Geometry check sheet. Reference: drawing and pictorial views, mm from the part's lowest x, y, z. Give positions to 0.01 mm unless a question says otherwise; leave off trailing zeros. Order: outer loops, then holes, each group sorted by start corner. A loop starts at its lowest first (then second) coordinate and runs counter-clockwise, first axis right, second up. Notation, with made-up numbers: M 89,43 L 146,43 A26 ccw 146,68 Z; hole C 80,40 d7. An arc over 180 degrees is marked long. Answer as a JSON object with one key per item and string values. Group by question number.
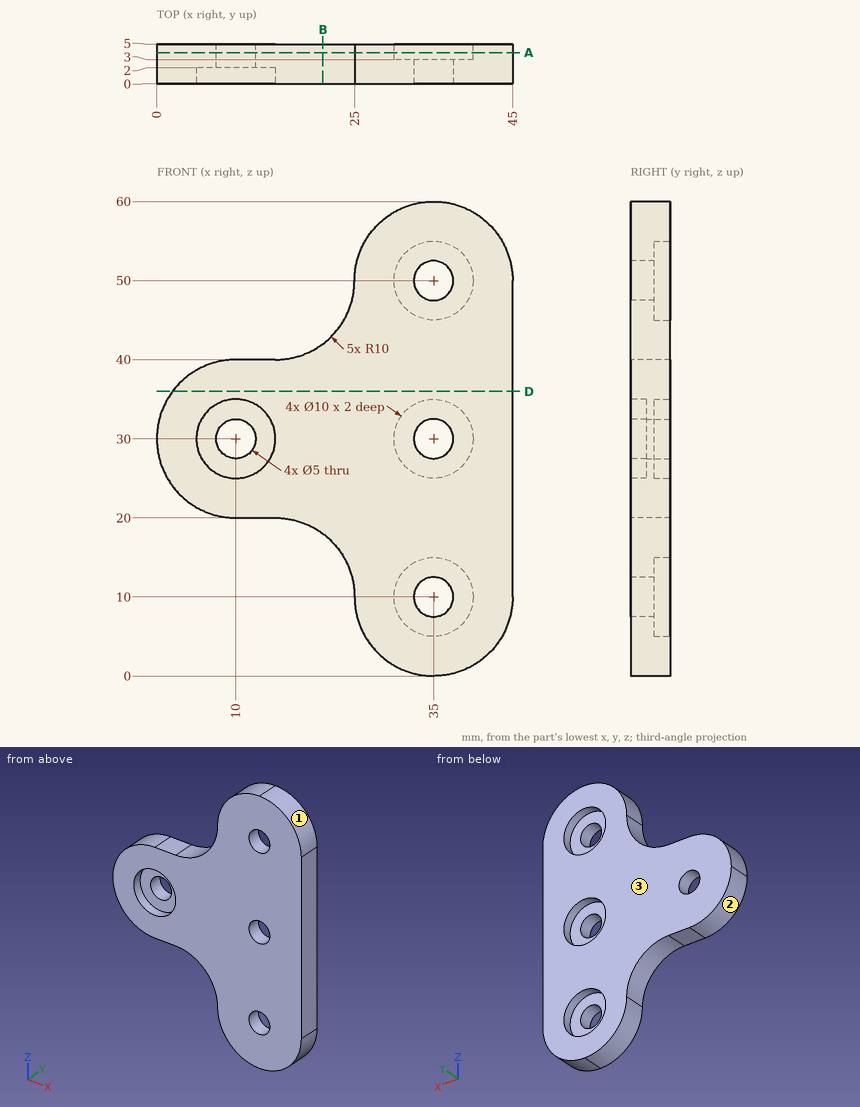
1. Thickness scan on line 1 along Z through (x, y) = (35, 1.65); line 2 along X through (y, z) = (0.85, 50); line 3 along Z through (x, y) = (35.5, 3.55). Record the ranges inside material, lowest first. Write a range as [from, to].
2. Depth check by flat-ended pin: pin 1 (6 mm diameter, centred on x = 35, z = 10, fed in from +Y); pin 2 (3 mm diameter, centred on x = 38.5, y = 1.5, fed in from +Z); pin 3 (2.5 mm diameter, centred on x = 12.5, y = 3.5, fed in from -Z). Enter the tip coordinate at first touch or a pass-through.
3. Cross-section at B-B (x = 21). Record the cut outline in (y, z), and give its area (3 significant figures).
4. Cross-section at A-A (y = 3.9). State how many separate pieces and enclosed holes the cut face has, and give its area (3 significant figures).
5. Release check for a two-part mould opening along Z. For the marked faces 1, 2 and 3 record: released by +Z, released by -Z, zero draft, split by the parting line, or undercut.
6. Cross-section at D-D (z = 36). Record the cut outline in (x, y), and give its area (3 significant figures).
Report:
{
 "1": {"line 1": "z = [0, 7.5], [12.5, 27.5], [32.5, 47.5], [52.5, 60]", "line 2": "x = [25, 32.5], [37.5, 45]", "line 3": "z = [0.01, 5.03], [14.97, 25.03], [34.97, 45.03], [54.97, 59.99]"},
 "2": {"pin 1": "stops at y = 3", "pin 2": "stops at z = 59.8", "pin 3": "stops at z = 20"},
 "3": {"outline": "M 0,18 L 5,18 L 5,42 L 0,42 Z", "area": "120 mm2"},
 "4": {"separate pieces": "1", "enclosed holes": "4", "area": "1,360 mm2"},
 "5": {"face 1": "released by +Z", "face 2": "released by -Z", "face 3": "zero draft"},
 "6": {"outline": "M 2,0 L 45,0 L 45,5 L 2,5 Z", "area": "215 mm2"}
}
